Build history of the part. All positions in model axes, mm. Face numbers are marked on the shaded views. A direction names the side the tool comes from. Round coordinates to 2 decimals unless told otherwise and drop trailing zeros. Write each loop counter-clockwise with the first axis right and the second up, starting at its lowest first coordinate (ties: lowest second). Pieces come first, ordered by that corner, then holes. Notation, with made-up numbers: (65.5, 78.5) - (101.5, 78.5) arc R28 ccw to (101.5, 111.5) - close; hole circle Ø11 at (56, -10). An arc over 180 degrees is marked (long way). One line per question, with ' | ' between items.
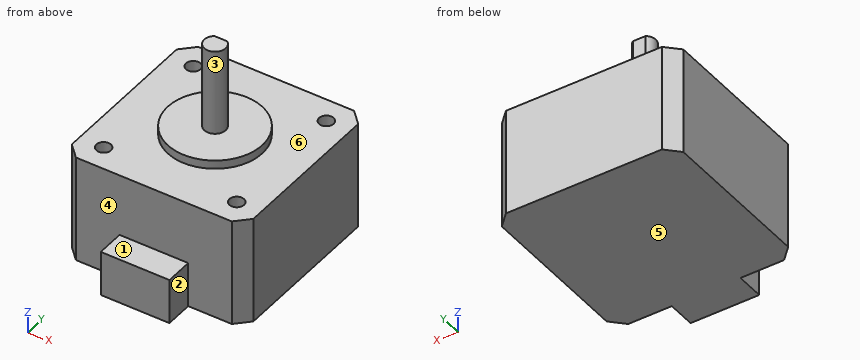
Autodesk Fusion 360 part; units mm, degrees
sketch "Esquisse1" plane through (0, 0, 0) normal (0, 0, 1) x (1, 0, 0)
  line L0 (21.15, 21.15) -> (-21.15, 21.15)
  line L1 (-21.15, 21.15) -> (-21.15, -21.15)
  line L2 (-21.15, -21.15) -> (21.15, -21.15)
  line L3 (21.15, -21.15) -> (21.15, 21.15)
  line L4 (21.15, 21.15) -> (-21.15, -21.15) construction
  line L5 (-21.15, 21.15) -> (21.15, -21.15) construction
  dimension "d1" = 42.3
  dimension "d2" = 42.3
extrude "Extrusion1" add sketch "Esquisse1" along normal blind 25
sketch "Esquisse2" plane through (0, 0, 25) normal (0, 0, 1) x (-1, 0, 0)
  line L0 (-21.15, 21.15) -> (-21.15, -21.15)
  line L1 (-21.15, -21.15) -> (21.15, -21.15)
  line L2 (21.15, -21.15) -> (21.15, 21.15)
  line L3 (21.15, 21.15) -> (-21.15, 21.15)
  circle A0 centre (15.5, -15.5) radius 1.7
  circle A1 centre (-15.5, -15.5) radius 1.7
  circle A2 centre (15.5, 15.5) radius 1.7
  circle A3 centre (-15.5, 15.5) radius 1.7
  dimension "d5" = 3.4
  dimension "d6" = 3.4
  dimension "d7" = 3.4
  dimension "d8" = 3.4
  dimension "d9" = 5.65
  dimension "d10" = 5.65
  dimension "d11" = 5.65
  dimension "d12" = 5.65
  dimension "d13" = 5.65
  dimension "d14" = 5.65
  dimension "d15" = 5.65
  dimension "d16" = 5.65
extrude "Extrusion2" cut sketch "Esquisse2" against normal blind 13.5 contours A0 | A1 | A2 | A3
sketch "Esquisse3" plane through (0, 0, 25) normal (0, 0, 1) x (-1, 0, 0)
  circle A0 centre (-15.5, -15.5) radius 1.7
  circle A1 centre (-15.5, 15.5) radius 1.7
  circle A2 centre (15.5, -15.5) radius 1.7
  circle A3 centre (15.5, 15.5) radius 1.7
  line L0 (-21.15, 21.15) -> (-21.15, -21.15)
  line L1 (-21.15, -21.15) -> (21.15, -21.15)
  line L2 (21.15, -21.15) -> (21.15, 21.15)
  line L3 (21.15, 21.15) -> (-21.15, 21.15)
  circle A4 centre (0, 0) radius 11
  circle A5 centre (0, 0) radius 2.5
  dimension "d19" = 22
  dimension "d20" = 5
extrude "Extrusion3" add sketch "Esquisse3" along normal blind 22 contours A5
extrude "Extrusion4" add sketch "Esquisse3" along normal blind 2 contours A4
sketch "Esquisse4" plane through (0, 0, 47) normal (0, 0, 1) x (-1, 0, 0)
  circle A0 centre (0, 0) radius 2.5
  line L0 (1.5, -2) -> (-1.5, -2)
  circle A1 centre (0, 0) radius 2.5
  dimension "d25" = 2
extrude "Extrusion5" cut sketch "Esquisse4" against normal blind 15 contours A0 L0 A1 picked at (-0.3999, -2.0645)
sketch "Esquisse5" plane through (0, 0, 0) normal (0, 0, -1) x (1, 0, 0)
  line L0 (21.15, -21.15) -> (21.15, 21.15)
  line L1 (21.15, 21.15) -> (-21.15, 21.15)
  line L2 (-21.15, 21.15) -> (-21.15, -21.15)
  line L3 (-21.15, -21.15) -> (21.15, -21.15)
  line L4 (8, 21.15) -> (-8, 21.15)
  line L5 (-8, 21.15) -> (-8, 27.65)
  line L6 (-8, 27.65) -> (8, 27.65)
  line L7 (8, 27.65) -> (8, 21.15)
  line L8 (8, 21.15) -> (-8, 27.65) construction
  line L9 (-8, 21.15) -> (8, 27.65) construction
  point P0 (0, 24.4)
  dimension "d28" = 6.5
  dimension "d29" = 16
  dimension "d30" = 13.15
extrude "Extrusion6" add sketch "Esquisse5" against normal blind 10.5 contours L1 L4 L5 L6 L7
chamfer "Chanfrein1" distance 3 angle 45 4 edges at (21.15, 21.15, 12.5) (21.15, -21.15, 12.5) (-21.15, 21.15, 12.5) (-21.15, -21.15, 12.5)
Q1. Saw through at D-D, the plane x = 0. List the corners of the cut face in (y, z), then the cut area to 3 significant figures.
Found:
outline: (-27.65, 0) - (21.15, 0) - (21.15, 25) - (11, 25) - (11, 27) - (2.5, 27) - (2.5, 32) - (2, 32) - (2, 47) - (-2.5, 47) - (-2.5, 27) - (-11, 27) - (-11, 25) - (-21.15, 25) - (-21.15, 10.5) - (-27.65, 10.5) - close | area: 1,260 mm^2
Q2. Which spindle directions (+Z, -Z, +X, -X, +Y, -Y) get a long thin tool onto all of the face, cutting with end or side? Do the marked faces 1, 2 and 3. Say none if no direction does.
Found:
face 1: +Z, +X, -X, -Y | face 2: +Z, -Z, +X, -Y | face 3: +Z
Q3. Pull direction Z, two halves, no side cores. Call the marked faces 4, 5 and 6: +Z half, -Z half, draft (parallel to the pull), parting line (faces both ways), or undercut.
Found:
face 4: draft | face 5: -Z half | face 6: +Z half
Q4. Saw through at A-A, the plane x = 15.5. List the corners of the cut face in (y, z).
Found:
outline: (-21.15, 0) - (21.15, 0) - (21.15, 25) - (17.2, 25) - (17.2, 11.5) - (13.8, 11.5) - (13.8, 25) - (-13.8, 25) - (-13.8, 11.5) - (-17.2, 11.5) - (-17.2, 25) - (-21.15, 25) - close
Q5. Drop flat-ended pins along their axis: pin 1 (3.5 mm diameter, centred on x = -14.5, y = 16, fed in from +Z); pin 2 (2 mm diameter, centred on y = -23, z = 4, fed in from -X); pin 3 (8 mm diameter, centred on x = 15.5, z = 12.5, fed in from -Y); pin 4 (1 mm diameter, centred on x = -4, z = 33.5, fed in from +Y). Give the stop position or say it passes through.
Found:
pin 1: z = 25 | pin 2: x = -8 | pin 3: y = -21.15 | pin 4: through
Q6. Saw through at C-C, the plane y = 10. List the corners of the cut face in (x, z), then the cut area to 3 significant figures.
Found:
outline: (-21.15, 0) - (21.15, 0) - (21.15, 25) - (4.58, 25) - (4.58, 27) - (-4.58, 27) - (-4.58, 25) - (-21.15, 25) - close | area: 1,080 mm^2
Q7. Saw through at B-B, the plane z = 8. List the corners of the cut face in (x, y).
Found:
outline: (-21.15, -18.15) - (-18.15, -21.15) - (-8, -21.15) - (-8, -27.65) - (8, -27.65) - (8, -21.15) - (18.15, -21.15) - (21.15, -18.15) - (21.15, 18.15) - (18.15, 21.15) - (-18.15, 21.15) - (-21.15, 18.15) - close
Q8. Drill centre lines: L1, parallel to X at y = -15.5, z = 20.25; L2, parallel to X at y = 15, z = 15. Where is each one in solid material? Low to high. Write a range as from..to.
Found:
L1: -21.15..-17.2, -13.8..13.8, 17.2..21.15 | L2: -21.15..-17.12, -13.88..13.88, 17.12..21.15
